Verification items for this drawing (mm, ordinates from the low corner). A direction names the side the tool comes from. Round coordinates to 2 decimals unless told otherwise and drop trailing zeros. Order: outer loops, then holes, each group sorted by start corner. A loop starts at its lowest first (then second) coordinate and runs counter-clockwise, first axis right, second up.
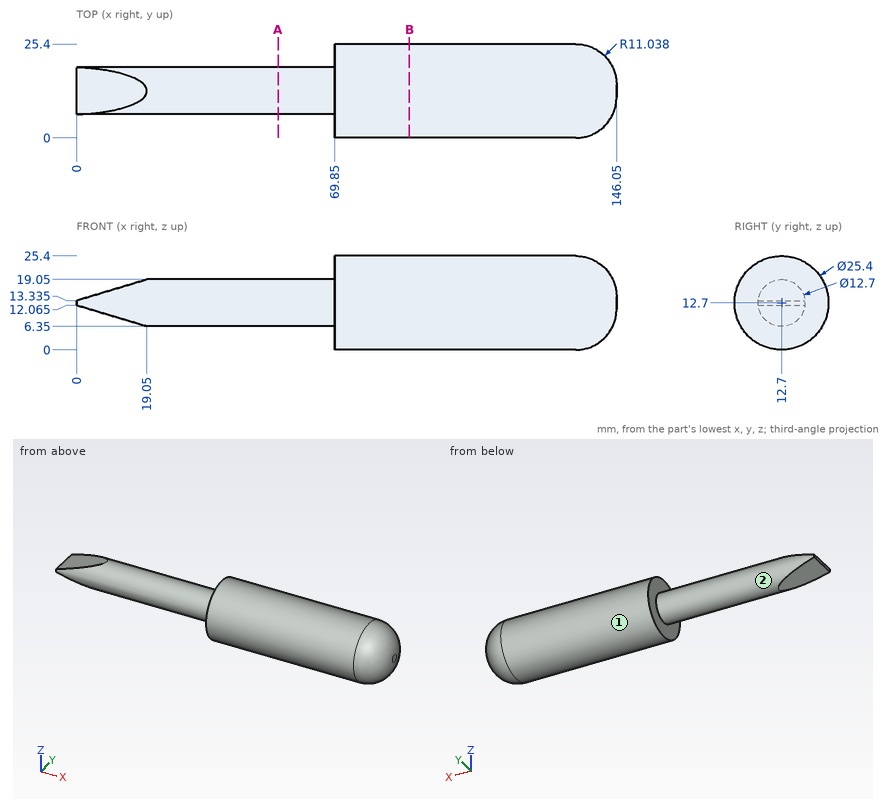
Item 1: Sectioned sample at A-A (x = 54.5). Record the cut outline in (y, z), and give its area (3 significant figures).
Answer:
outline: circle Ø12.7 at (12.7, 12.7)
area: 127 mm2
Item 2: Access from +Z, -Z, +X, -X, +Y, -Y to the whole of each face (thin tool, end or side, straight path). Record for the marked faces 1 and 2.
Answer:
face 1: +X, -X
face 2: -X
Item 3: Go/stop test with flat-tipped pins: P1, Ø3, axis at x = 71.5, y = 10, coming from the -Z side; P2, Ø3, axis at y = 9, z = 20, coming from the +X side; P3, Ø1, axis at x = 31, z = 18, coming from the +Y side. Record where each tip stops, or that it passes through.
Answer:
P1: stops at z = 0.06
P2: stops at x = 144.84
P3: stops at y = 16.86
Item 4: Sectioned sample at B-B (x = 90). Record the cut outline in (y, z).
Answer:
outline: circle Ø25.4 at (12.7, 12.7)
Item 5: Scan lines: line 1 along Y through (x, z) = (116.5, 13.25); line 2 along Y through (x, z) = (120, 10.25); line 3 along Z through (x, y) = (61, 11.75). Record each from-to range of solid material in increasing order.
Answer:
line 1: y = 0.01 to 25.39
line 2: y = 0.24 to 25.16
line 3: z = 6.42 to 18.98
